Model file for the job. Use its own axes, mm. A direction names the side the tool comes from. Give positions to 0.01 mm unless a question says otherwise; leave off trailing zeros. Loops run counter-clockwise (first coordinate to the right, second up) from the corner with the lowest first, then second, coordinate; pieces in that order, holes last. Notation, with made-up numbers: M -23.75,3 L -10.75,3 A30 ccw -10.75,34 Z; hole C 1,89 d9. An arc over 180 degrees is marked long. Use CSV: the item, a comma, the result in double quotes. Start each with the question number.
(1) Tool access for faces 4 (the face through (42, -5, 13.5)), 5 (the face through (17, -5, 18)), 6 (the face through (3, -7, 8)): list every direction of +Z, -Z, +X, -X, +Y, -Y with a clear straight run to the whole face (end or side of a thin tool).
(2) Slice it at C-C on z = 2. List the corners of the cut face in (x, y), and give its area (3 significant figures).
(3) Slice it at A-A on x = 45.5. List the corners of the cut face in (y, z).
(4) Two-plate mould, pull along X, no slides. Class faces 1 (the face through (35, -5, 7)), 2 (the face through (8, -5, 15)), 3 (the face through (47.81, -5.96, 16.8)): pulls with the +X half, pulls with the -X half, needs draft (parallel to the pull), parting line crosses it, or undercut.
(5) Slice it at B-B on y = -5. List the corners of the cut face in (x, z).
(6) Flat gauge pins, fed straight in: P1, Ø5, axis at x = 3, y = -5, coming from the -Z side; P2, Ø5, axis at y = -8.5, z = 9.5, coming from the +X side; P3, Ø3, axis at x = 41.5, y = -3, coming from the -Z side; P4, Ø3, axis at x = 7, y = -6.5, coming from the +Z side. Where does each tip first touch, or does it go through?
(7) Slice it at D-D on z = 16.5. List the corners of the cut face in (x, y), and give its area (3 significant figures).
(8) Wall check: line 1 along Y through (x, z) = (45.5, 18); line 2 along Z through (x, y) = (6, -4.5); line 3 along Y through (x, z) = (14, 10). Give the ranges that are in metal, low to high. Write a range as from..to.
```python
from build123d import *

# Parameters (mm, degrees)
ESQUISSE1_W      = 52.5
ESQUISSE1_H      = 10
EXTRUSION1_DEPTH = 20
ESQUISSE3_R      = 2
EXTRUSION3_DEPTH = 21
ESQUISSE4_R      = 2.5
EXTRUSION4_DEPTH = 20
ESQUISSE2_W      = 17
ESQUISSE2_H      = 5
ESQUISSE2_W_2    = 17.5
ESQUISSE2_H_2    = 13.5
EXTRUSION5_DEPTH = 20


with BuildPart() as part:
    # Esquisse1 → Extrusion1 (new body)
    with BuildSketch(Plane.XY):
        with Locations((26.25, -5)):
            Rectangle(ESQUISSE1_W, ESQUISSE1_H)
    extrude(amount=EXTRUSION1_DEPTH)

    # Esquisse3 → Extrusion3 (cut, through all)
    with BuildSketch(Plane.XY.offset(20)):
        with Locations((3, -5)):
            Circle(ESQUISSE3_R)
        with Locations((14, -5)):
            Circle(ESQUISSE3_R)
    extrude(amount=-EXTRUSION3_DEPTH, mode=Mode.SUBTRACT)

    # Esquisse4 → Extrusion4 (cut)
    with BuildSketch(Plane.XY.offset(20)):
        with Locations((45.5, -5)):
            Circle(ESQUISSE4_R)
    extrude(amount=-EXTRUSION4_DEPTH, mode=Mode.SUBTRACT)

    # Esquisse2 → Extrusion5 (cut)
    with BuildSketch(Plane(origin=(0, 0, 0), x_dir=(1, 0, 0), z_dir=(0, 1, 0))):
        with Locations((8.5, -17.5)):
            Rectangle(ESQUISSE2_W, ESQUISSE2_H)
        with Locations((43.75, -6.75)):
            Rectangle(ESQUISSE2_W_2, ESQUISSE2_H_2)
    extrude(amount=-EXTRUSION5_DEPTH, mode=Mode.SUBTRACT)


solid = part.part
```
Reply:
1,face 4,"-Z, +X, +Y, -Y"
1,face 5,"+Z, -X, +Y, -Y"
1,face 6,"+Z, -Z"
2,outline,"M 0,-10 L 35,-10 L 35,0 L 0,0 Z; hole C 3,-5 d4; hole C 14,-5 d4"
2,area,"325 mm^2"
3,outline,"M -10,13.5 L -7.5,13.5 L -7.5,20 L -10,20 Z; M -2.5,13.5 L 0,13.5 L 0,20 L -2.5,20 Z"
4,face 1,"pulls with the +X half"
4,face 2,"needs draft"
4,face 3,"undercut"
5,outline,"M 0,0 L 1,0 L 1,15 L 0,15 Z; M 5,0 L 12,0 L 12,15 L 5,15 Z; M 16,0 L 35,0 L 35,13.5 L 43,13.5 L 43,20 L 17,20 L 17,15 L 16,15 Z; M 48,13.5 L 52.5,13.5 L 52.5,20 L 48,20 Z"
6,P1,"stops at z = 0"
6,P2,"stops at x = 35"
6,P3,"stops at z = 13.5"
6,P4,"stops at z = 15"
7,outline,"M 17,-10 L 52.5,-10 L 52.5,0 L 17,0 Z; hole C 45.5,-5 d5"
7,area,"335 mm^2"
8,line 1,"y = -10..-7.5, -2.5..0"
8,line 2,"z = 0..15"
8,line 3,"y = -10..-7, -3..0"
